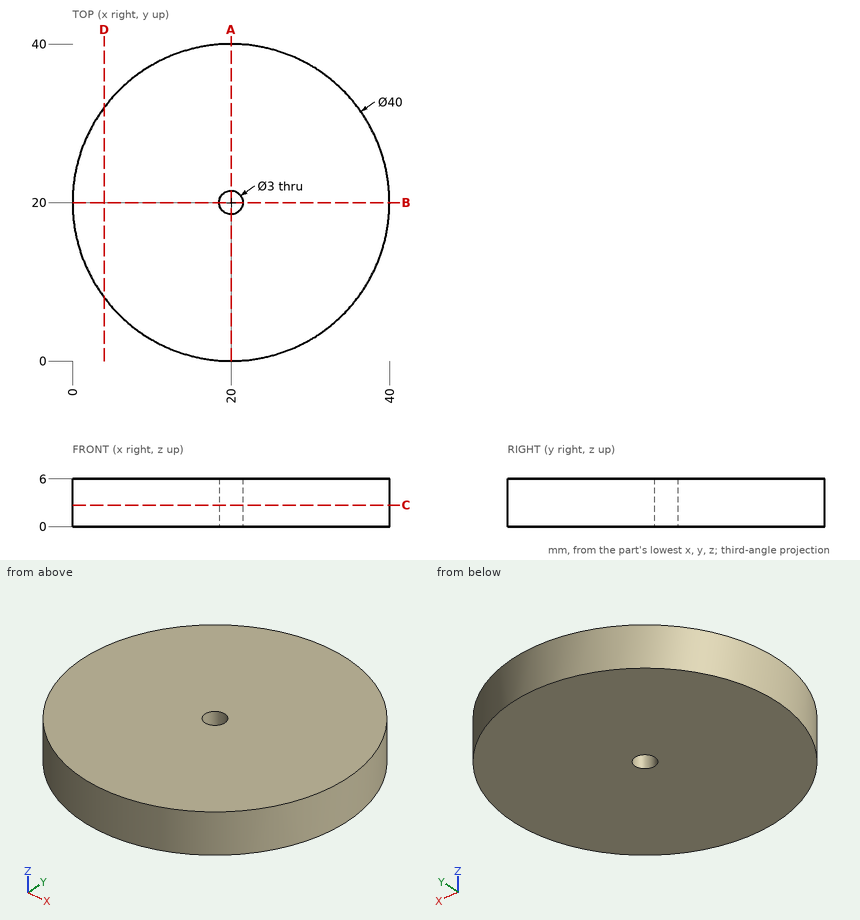
Study the drawing (mm; zero at the part's minimum x, y, z) and answer. Coordinates: 2 decimals unless noted, no trailing zeros. Write each loop counter-clockwise with the first axis right and the second up, starting at its lowest first coordinate (ties: lowest second). Pieces come first, ordered by that corner, then holes. Notation, with made-up numbers: (42.25, -29.5) - (47.25, -29.5) arc R20 cw to (47.25, -21.5) - close; hole circle Ø5 at (10, 69). An arc over 180 degrees is marked (long way). Return JSON: item names as keys, results as strings. Group by question number.
1. A cutting plane is placed at C-C, the plane z = 2.7. Determine the outline of the cut face in (x, y).
2. A cutting plane is placed at D-D, the plane x = 4. Determine the outline of the cut face in (y, z).
3. Given pin 1 (2 mm diameter, centred on x = 27, z = 4.5, fed in from -Y), flat-ended and moving along its own axis, determine where the tip first touches the part or whether it passes through.
4. Straight lines are drawn through the part: L1, parallel to Y at x = 20, z = 1.3; L2, parallel to Y at x = 13, z = 2.55 (3 decimals); L3, parallel to X at y = 20.5, z = 1.45. For each, find the intervals that lie inside material, in ascending order.
5. A cutting plane is placed at A-A, the plane x = 20. Determine the outline of the cut face in (y, z).
Ans:
{
 "1": {"outline": "circle Ø40 at (20, 20); hole circle Ø3 at (20, 20)"},
 "2": {"outline": "(8, 0) - (32, 0) - (32, 6) - (8, 6) - close"},
 "3": {"pin 1": "y = 0.92"},
 "4": {"L1": "0 to 18.5, 21.5 to 40", "L2": "1.265 to 38.735", "L3": "0.01 to 18.59, 21.41 to 39.99"},
 "5": {"outline": "(0, 0) - (18.5, 0) - (18.5, 6) - (0, 6) - close; (21.5, 0) - (40, 0) - (40, 6) - (21.5, 6) - close"}
}
